```python
from build123d import *

# Parameters (mm, degrees)
SKETCH2_W          = 0.6
SKETCH2_H          = 4.5
CUT_EXTRUDE1_DEPTH = 0.7


with BuildPart() as part:
    # Sketch1 → Revolve1 (revolve)
    with BuildSketch(Plane(origin=(0, 0, 0), x_dir=(0, 0, -1), z_dir=(1, 0, 0))):
        with BuildLine():
            Line((0, 0), (0, 2.018385021))
            ThreePointArc((0, 2.018385021), (0.026272266, 2.085944042), (0.091284426, 2.118004491))
            Line((0.091284426, 2.118004491), (1.6, 2.25))
            Line((1.6, 2.25), (1.6, 1.35))
            ThreePointArc((1.6, 1.35), (1.629289322, 1.279289322), (1.7, 1.25))
            Line((1.7, 1.25), (7.375, 1.25))
            Line((7.375, 1.25), (7.6, 1.025))
            Line((7.6, 1.025), (7.6, 0))
            Line((7.6, 0), (0, 0))
        make_face()
    revolve(axis=Axis((0, 0, 0), (0, 0, -1)))

    # Sketch2 → Cut-Extrude1 (cut)
    with BuildSketch(Plane.XY):
        Rectangle(SKETCH2_W, SKETCH2_H)
    extrude(amount=-CUT_EXTRUDE1_DEPTH, mode=Mode.SUBTRACT)


solid = part.part
```
Check sheet for the modelled part. Datum: model origin and axes. Units: mm. A direction names the side the tool comes from. Give positions to 0.01 mm unless a question says otherwise; leave off trailing zeros. Write each loop counter-clockwise with the first axis right and the second up, starting at its lowest first coordinate (ties: lowest second). Pieces come first, ordered by that corner, then holes. Notation, with made-up numbers: (23.25, 73) -> (29.25, 73) arc R19 cw to (29.25, 87) -> close; hole circle Ø2 at (62.25, -30.75). An arc over 180 degrees is marked (long way). Use CSV: the item, a comma, the result in double quotes. Start each with the question number.
Q1. Cross-section at A-A on y = 0. Enter the section's corners in (x, z) (3 decimals), and give its area (3 significant figures).
Q2. Cross-section at B-B on x = 0. Enter the section's corners in (y, z) (3 decimals), and give its area (3 significant figures).
Q3. Scan lines: line 1 along Z through (x, y) = (0.65, 1.9); line 2 along X through (y, z) = (-0.85, -0.25); line 3 along Z through (x, y) = (0, 0.9). Record each from-to range of solid material in increasing order.
Q4. Cross-section at C-C on z = -6. Enter the section's corners in (x, y), and give its area (3 significant figures).
Q5. Tool access check on faces 1 (the conical face through (-0.831, 2.005, -0.689)), 2 (the cylindrical face through (-1.22, -0.27, -4.58)). Record the directions out of +Z, -Z, +X, -X, +Y, -Y that give a thin tool (end or side, any length) a straight path to the whole face; none if there is none.
Q6. Depth check by flat-ended pin: P1, Ø1, axis at y = -2, z = -3, coming from the +X side; P2, Ø0.8, axis at y = 0.5, z = -0.5, coming from the +X side; P3, Ø0.5, axis at x = 0, y = -1, coming from the +Z side; P4, Ø1, axis at x = -1, y = -1, coming from the -Z side. Enter the tip coordinate at first touch or a pass-through.
Working result:
1,outline,"(-2.25, -1.6) -> (-1.35, -1.6) arc R0.1 cw to (-1.25, -1.7) -> (-1.25, -7.375) -> (-1.025, -7.6) -> (1.025, -7.6) -> (1.25, -7.375) -> (1.25, -1.7) arc R0.1 cw to (1.35, -1.6) -> (2.25, -1.6) -> (2.118, -0.091) arc R0.1 ccw to (2.018, 0) -> (0.3, 0) -> (0.3, -0.7) -> (-0.3, -0.7) -> (-0.3, 0) -> (-2.018, 0) arc R0.1 ccw to (-2.118, -0.091) -> close"
1,area,"21.5 mm^2"
2,outline,"(-2.25, -1.6) -> (-1.35, -1.6) arc R0.1 cw to (-1.25, -1.7) -> (-1.25, -7.375) -> (-1.025, -7.6) -> (1.025, -7.6) -> (1.25, -7.375) -> (1.25, -1.7) arc R0.1 cw to (1.35, -1.6) -> (2.25, -1.6) -> (2.171, -0.7) -> (-2.171, -0.7) -> close"
2,area,"18.9 mm^2"
3,line 1,"z = -1.6 to 0"
3,line 2,"x = -1.96 to -0.3, 0.3 to 1.96"
3,line 3,"z = -7.6 to -0.7"
4,outline,"circle Ø2.5 at (0, 0)"
4,area,"4.91 mm^2"
5,face 1,"+Z"
5,face 2,"-Z"
6,P1,"passes through"
6,P2,"stops at x = 2.17"
6,P3,"stops at z = -0.7"
6,P4,"stops at z = -7.6"
